Check sheet for the modelled part. Datum: model origin and axes. Units: mm. A direction names the side the tool comes from. Round coordinates to 2 decimals unless told otherwise and drop trailing zeros. Order: outer loops, then holes, each group sorted by start corner. A loop starts at its lowest first (then second) coordinate and runs counter-clockwise, first axis right, second up. Notation, with made-up numbers: (-31.75, 6.25) -> (6.25, 6.25) arc R24 cw to (6.25, 24.25) -> close; hole circle Ø10 at (41.25, 81). An arc over 180 degrees is marked (long way). Answer in a Markdown table with one row per item.
from build123d import *

# Parameters (mm, degrees)
SKETCH1_R           = 5
SKETCH1_R_2         = 0.75
BOSS_EXTRUDE1_DEPTH = 3


with BuildPart() as part:
    # Sketch1 → Boss-Extrude1 (new body)
    with BuildSketch(Plane.XY):
        Polygon((-13.25, 15.5), (-10.25, 15.5), (-10.25, 10.5), (-13.25, 10.5), (-13.25, 5.35), (-10.25, 5.35), (-10.25, 0.35), (-13.25, 0.35), (-13.25, -4.65), (-10.25, -4.65), (-10.25, -9.65), (-13.25, -9.65), (-13.25, -20.5), (13.25, -20.5), (13.25, -9.65), (10.25, -9.65), (10.25, -4.65), (13.25, -4.65), (13.25, 0.35), (10.25, 0.35), (10.25, 5.35), (13.25, 5.35), (13.25, 10.5), (10.25, 10.5), (10.25, 15.5), (13.25, 15.5), (13.25, 20.5), (-13.25, 20.5), align=None)
        with Locations((0, 10.5)):
            Circle(SKETCH1_R, mode=Mode.SUBTRACT)
        with Locations((3.75, 16.995190528)):
            Circle(SKETCH1_R_2, mode=Mode.SUBTRACT)
        with Locations((7.499999997, 10.499776304)):
            Circle(SKETCH1_R_2, mode=Mode.SUBTRACT)
        with Locations((3.75, 4.004809472)):
            Circle(SKETCH1_R_2, mode=Mode.SUBTRACT)
        with Locations((-3.75, 4.004809472)):
            Circle(SKETCH1_R_2, mode=Mode.SUBTRACT)
        with Locations((-7.499999997, 10.500223696)):
            Circle(SKETCH1_R_2, mode=Mode.SUBTRACT)
        with Locations((-3.75, 16.995190528)):
            Circle(SKETCH1_R_2, mode=Mode.SUBTRACT)
    extrude(amount=BOSS_EXTRUDE1_DEPTH)


solid = part.part
Item 1: Cross-section at C-C (x = 3.75). Record the boundary of the cut face in (y, z).
Result sheet:
| item | result |
|---|---|
| outline | (-20.5, 0) -> (3.25, 0) -> (3.25, 3) -> (-20.5, 3) -> close; (4.75, 0) -> (7.19, 0) -> (7.19, 3) -> (4.75, 3) -> close; (13.81, 0) -> (16.25, 0) -> (16.25, 3) -> (13.81, 3) -> close; (17.75, 0) -> (20.5, 0) -> (20.5, 3) -> (17.75, 3) -> close |
Item 2: Scan lines: line 1 (Y direction, x = 10.5, z = 2.9); line 2 (X direction, y = 4, z = 2.1); line 3 (Y direction, x = -4.25, z = 2.85). Record each from-to range of solid material in increasing order. Write a range as [from, to].
Result sheet:
| item | result |
|---|---|
| line 1 | y = [-20.5, -9.65], [-4.65, 0.35], [5.35, 10.5], [15.5, 20.5] |
| line 2 | x = [-10.25, -4.5], [-3, 3], [4.5, 10.25] |
| line 3 | y = [-20.5, 3.45], [4.56, 7.87], [13.13, 16.44], [17.55, 20.5] |
Item 3: Depth check by flat-ended pin: P1, Ø0.9, axis at x = 3.75, y = 4, coming from the -Z side; P2, Ø1.5, axis at y = -8, z = 1.5, coming from the +X side. Enter the tip coordinate at first touch or a pass-through.
Result sheet:
| item | result |
|---|---|
| P1 | passes through |
| P2 | stops at x = 10.25 |
Item 4: Cross-section at B-B (y = 6.5). Record the boundary of the cut face in (x, z), and give its area (3 significant figures).
Result sheet:
| item | result |
|---|---|
| outline | (-13.25, 0) -> (-3, 0) -> (-3, 3) -> (-13.25, 3) -> close; (3, 0) -> (13.25, 0) -> (13.25, 3) -> (3, 3) -> close |
| area | 61.5 mm^2 |
Item 5: Mould release check, pull along Y, two halves, no side actions. Record for faces 1 (the flat face through (0, 0, 0)), 2 (the flat face through (0, -20.5, 1)), 3 (the cylindrical face through (3.65, 17.74, 1.48)): pulls with the +Y half, pulls with the -Y half, needs draft (parallel to the pull), parting line crosses it, or undercut.
Result sheet:
| item | result |
|---|---|
| face 1 | needs draft |
| face 2 | pulls with the -Y half |
| face 3 | undercut |
Item 6: Set-up check for faces 4 (the cylindrical face through (-6.785, 10.726, 1.479)), 5 (the flat face through (-10.25, -7, 1)), 6 (the flat face through (12, 15.5, 1)): record each of +Z, -Z, +X, -X, +Y, -Y from which the full face is reachable in a straight line by a thin tool's end or side.
Result sheet:
| item | result |
|---|---|
| face 4 | +Z, -Z |
| face 5 | +Z, -Z, -X |
| face 6 | +Z, -Z, +X |
Item 7: Cross-section at A-A (x = 0). Record the boundary of the cut face in (y, z).
Result sheet:
| item | result |
|---|---|
| outline | (-20.5, 0) -> (5.5, 0) -> (5.5, 3) -> (-20.5, 3) -> close; (15.5, 0) -> (20.5, 0) -> (20.5, 3) -> (15.5, 3) -> close |
Item 8: Cross-section at D-D (z = 1). State how many separate pieces and enclosed holes the cut face has, and give its area (3 significant figures).
Result sheet:
| item | result |
|---|---|
| separate pieces | 1 |
| enclosed holes | 7 |
| area | 907 mm^2 |
